Verification items for the finished model (mm, model axes). Face numbers are marked on the shaded views. A direction names the side the tool comes from. Round coordinates to 2 decimals unless told otherwise and drop trailing zeros. Write each loop counter-clockwise with the first axis right and the second up, starting at its lowest first coordinate (ties: lowest second). Pieces come first, ordered by that corner, then holes. Notation, with made-up numbers: (7.25, -29.75) - (21.25, -29.75) arc R33 ccw to (21.25, 2.25) - close; hole circle Ø6 at (7.25, -16.75). An arc over 180 degrees is marked (long way). Answer as a JSON object with one key per item and string values.
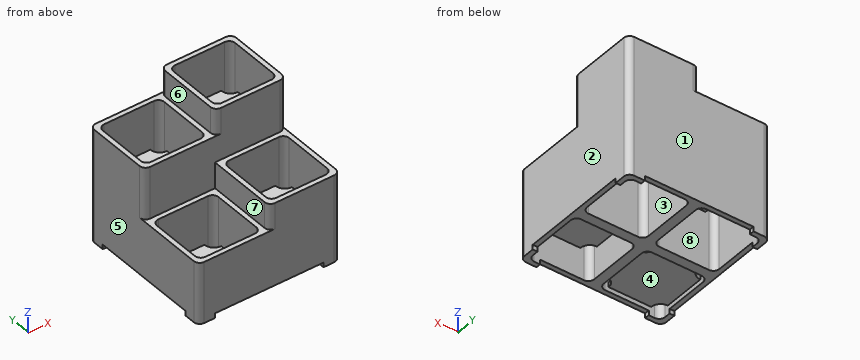
```python
from build123d import *

# Parameters (mm, degrees)
F0_W      = 4
F0_H      = 4
F1_DEPTH  = 48
F2_DEPTH  = 8
F3_DEPTH  = 70
F4_DEPTH  = 30
F0_H_2    = 23.163830772
F5_DEPTH  = 114
F6_DEPTH  = 74
F0_W_2    = 10.0586636961
F7_DEPTH  = 92
F8_DEPTH  = 52
F9_DEPTH  = 4
F10_DEPTH = 48
F11_DEPTH = 26
F12_DEPTH = 70
F13_DEPTH = 4
F14_R     = 5


with BuildPart() as f1:
    # F0 (on Top) → F1 (new body)
    with BuildSketch(Plane.XY):
        Polygon((-12, -4), (-4, -4), (-4, 0), (-56, 0), (-56, -4), (-48, -4), align=None)
        Polygon((-60, -56), (-56, -56), (-56, -48), (-56, -46), (-60, -46), align=None)
        Polygon((-4, -56), (0, -56), (0, -4), (-4, -4), (-4, -12), (-4, -48), align=None)
        with Locations((-2, -2)):
            Rectangle(F0_W, F0_H)
        Polygon((-60, 0), (-60, -46), (-56, -46), (-56, -16.2410065532), (-56, -12), (-56, -4), (-56, 0), align=None)
        Polygon((-46, -60), (0, -60), (0, -56), (-4, -56), (-12, -56), (-46, -56), align=None)
        Polygon((-56, -60), (-46, -60), (-46, -56), (-48, -56), (-56, -56), align=None)
        with Locations((-58, -58)):
            Rectangle(F0_W, F0_H)
    extrude(amount=F1_DEPTH)

    # F0 (on Top) → F2 (join)
    with BuildSketch(Plane.XY):
        with BuildLine():
            Line((-48, -56), (-46, -56))
            Line((-46, -56), (-12, -56))
            ThreePointArc((-12, -56), (-9.6568542495, -50.3431457505), (-4, -48))
            Line((-4, -48), (-4, -12))
            ThreePointArc((-4, -12), (-9.6568542495, -9.6568542495), (-12, -4))
            Line((-12, -4), (-48, -4))
            ThreePointArc((-48, -4), (-50.3431457505, -9.6568542495), (-56, -12))
            Line((-56, -12), (-56, -16.2410065532))
            Line((-56, -16.2410065532), (-56, -46))
            Line((-56, -46), (-56, -48))
            ThreePointArc((-56, -48), (-50.3431457505, -50.3431457505), (-48, -56))
        make_face()
    extrude(amount=F2_DEPTH)

    # F0 (on Top) → F3 (join)
    with BuildSketch(Plane.XY):
        Polygon((0, -4), (0, -56), (4, -56), (4, -48), (4, -12), (4, -4), align=None)
        with Locations((2, -2)):
            Rectangle(F0_W, F0_H)
        Polygon((56, -4), (56, 0), (4, 0), (4, -4), (12, -4), (48, -4), align=None)
        Polygon((56, -46), (60, -46), (60, 0), (56, 0), (56, -4), (56, -12), align=None)
        Polygon((0, -60), (46, -60), (46, -56), (12, -56), (4, -56), (0, -56), align=None)
        Polygon((56, -56), (60, -56), (60, -46), (56, -46), (56, -48), align=None)
        with Locations((58, -58)):
            Rectangle(F0_W, F0_H)
        Polygon((46, -60), (56, -60), (56, -56), (48, -56), (46, -56), align=None)
    extrude(amount=F3_DEPTH)

    # F0 (on Top) → F4 (join)
    with BuildSketch(Plane.XY):
        with BuildLine():
            Line((12, -56), (46, -56))
            Line((46, -56), (48, -56))
            ThreePointArc((48, -56), (50.3431457505, -50.3431457505), (56, -48))
            Line((56, -48), (56, -46))
            Line((56, -46), (56, -12))
            ThreePointArc((56, -12), (50.3431457505, -9.6568542495), (48, -4))
            Line((48, -4), (12, -4))
            ThreePointArc((12, -4), (9.6568542495, -9.6568542495), (4, -12))
            Line((4, -12), (4, -48))
            ThreePointArc((4, -48), (9.6568542495, -50.3431457505), (12, -56))
        make_face()
    extrude(amount=F4_DEPTH)

    # F0 (on Top) → F5 (join)
    with BuildSketch(Plane.XY):
        Polygon((0, 4), (4, 4), (4, 12), (4, 48), (4, 56), (0, 56), align=None)
        Polygon((0, 60), (0, 56), (4, 56), (12, 56), (46, 56), (46, 60), align=None)
        with Locations((58, 34.418084614)):
            Rectangle(F0_W, F0_H_2)
        Polygon((56, 0), (60, 0), (60, 22.836169228), (56, 22.836169228), (56, 12), (56, 4), align=None)
        Polygon((4, 0), (56, 0), (56, 4), (48, 4), (12, 4), (4, 4), align=None)
        with Locations((2, 2)):
            Rectangle(F0_W, F0_H)
        Polygon((48, 56), (56, 56), (56, 60), (46, 60), (46, 56), align=None)
        with Locations((58, 58)):
            Rectangle(F0_W, F0_H)
        Polygon((56, 46), (60, 46), (60, 56), (56, 56), (56, 48), align=None)
    extrude(amount=F5_DEPTH)

    # F0 (on Top) → F6 (join)
    with BuildSketch(Plane.XY):
        with BuildLine():
            Line((56, 12), (56, 22.836169228))
            Line((56, 22.836169228), (56, 46))
            Line((56, 46), (56, 48))
            ThreePointArc((56, 48), (50.3431457505, 50.3431457505), (48, 56))
            Line((48, 56), (46, 56))
            Line((46, 56), (12, 56))
            ThreePointArc((12, 56), (9.6568542495, 50.3431457505), (4, 48))
            Line((4, 48), (4, 12))
            ThreePointArc((4, 12), (9.6568542495, 9.6568542495), (12, 4))
            Line((12, 4), (48, 4))
            ThreePointArc((48, 4), (50.3431457505, 9.6568542495), (56, 12))
        make_face()
    extrude(amount=F6_DEPTH)

    # F0 (on Top) → F7 (join)
    with BuildSketch(Plane.XY):
        Polygon((-56, 0), (-4, 0), (-4, 4), (-12, 4), (-48, 4), (-56, 4), align=None)
        Polygon((-4, 4), (0, 4), (0, 56), (-4, 56), (-4, 48), (-4, 12), align=None)
        with Locations((-2, 2)):
            Rectangle(F0_W, F0_H)
        Polygon((-4, 56), (0, 56), (0, 60), (-35.9413363039, 60), (-35.9413363039, 56), (-12, 56), align=None)
        with Locations((-40.970668152, 58)):
            Rectangle(F0_W_2, F0_H)
        Polygon((-60, 0), (-56, 0), (-56, 4), (-56, 12), (-56, 46), (-60, 46), align=None)
        Polygon((-46, 56), (-46, 60), (-56, 60), (-56, 56), (-48, 56), align=None)
        with Locations((-58, 58)):
            Rectangle(F0_W, F0_H)
        Polygon((-60, 56), (-60, 46), (-56, 46), (-56, 48), (-56, 56), align=None)
    extrude(amount=F7_DEPTH)

    # F0 (on Top) → F8 (join)
    with BuildSketch(Plane.XY):
        with BuildLine():
            ThreePointArc((-12, 4), (-9.6568542495, 9.6568542495), (-4, 12))
            Line((-4, 12), (-4, 48))
            ThreePointArc((-4, 48), (-9.6568542495, 50.3431457505), (-12, 56))
            Line((-12, 56), (-35.9413363039, 56))
            Line((-35.9413363039, 56), (-46, 56))
            Line((-46, 56), (-48, 56))
            ThreePointArc((-48, 56), (-50.3431457505, 50.3431457505), (-56, 48))
            Line((-56, 48), (-56, 46))
            Line((-56, 46), (-56, 12))
            ThreePointArc((-56, 12), (-50.3431457505, 9.6568542495), (-48, 4))
            Line((-48, 4), (-12, 4))
        make_face()
    extrude(amount=F8_DEPTH)

    # F0 (on Top) → F9 (cut)
    with BuildSketch(Plane.XY):
        with BuildLine():
            Line((-48, -56), (-46, -56))
            Line((-46, -56), (-12, -56))
            ThreePointArc((-12, -56), (-9.6568542495, -50.3431457505), (-4, -48))
            Line((-4, -48), (-4, -12))
            ThreePointArc((-4, -12), (-9.6568542495, -9.6568542495), (-12, -4))
            Line((-12, -4), (-48, -4))
            ThreePointArc((-48, -4), (-50.3431457505, -9.6568542495), (-56, -12))
            Line((-56, -12), (-56, -16.2410065532))
            Line((-56, -16.2410065532), (-56, -46))
            Line((-56, -46), (-56, -48))
            ThreePointArc((-56, -48), (-50.3431457505, -50.3431457505), (-48, -56))
        make_face()
    extrude(amount=F9_DEPTH, mode=Mode.SUBTRACT)

    # F0 (on Top) → F10 (cut)
    with BuildSketch(Plane.XY):
        with BuildLine():
            ThreePointArc((-12, 4), (-9.6568542495, 9.6568542495), (-4, 12))
            Line((-4, 12), (-4, 48))
            ThreePointArc((-4, 48), (-9.6568542495, 50.3431457505), (-12, 56))
            Line((-12, 56), (-35.9413363039, 56))
            Line((-35.9413363039, 56), (-46, 56))
            Line((-46, 56), (-48, 56))
            ThreePointArc((-48, 56), (-50.3431457505, 50.3431457505), (-56, 48))
            Line((-56, 48), (-56, 46))
            Line((-56, 46), (-56, 12))
            ThreePointArc((-56, 12), (-50.3431457505, 9.6568542495), (-48, 4))
            Line((-48, 4), (-12, 4))
        make_face()
    extrude(amount=F10_DEPTH, mode=Mode.SUBTRACT)

    # F0 (on Top) → F11 (cut)
    with BuildSketch(Plane.XY):
        with BuildLine():
            Line((12, -56), (46, -56))
            Line((46, -56), (48, -56))
            ThreePointArc((48, -56), (50.3431457505, -50.3431457505), (56, -48))
            Line((56, -48), (56, -46))
            Line((56, -46), (56, -12))
            ThreePointArc((56, -12), (50.3431457505, -9.6568542495), (48, -4))
            Line((48, -4), (12, -4))
            ThreePointArc((12, -4), (9.6568542495, -9.6568542495), (4, -12))
            Line((4, -12), (4, -48))
            ThreePointArc((4, -48), (9.6568542495, -50.3431457505), (12, -56))
        make_face()
    extrude(amount=F11_DEPTH, mode=Mode.SUBTRACT)

    # F0 (on Top) → F12 (cut)
    with BuildSketch(Plane.XY):
        with BuildLine():
            Line((56, 12), (56, 22.836169228))
            Line((56, 22.836169228), (56, 46))
            Line((56, 46), (56, 48))
            ThreePointArc((56, 48), (50.3431457505, 50.3431457505), (48, 56))
            Line((48, 56), (46, 56))
            Line((46, 56), (12, 56))
            ThreePointArc((12, 56), (9.6568542495, 50.3431457505), (4, 48))
            Line((4, 48), (4, 12))
            ThreePointArc((4, 12), (9.6568542495, 9.6568542495), (12, 4))
            Line((12, 4), (48, 4))
            ThreePointArc((48, 4), (50.3431457505, 9.6568542495), (56, 12))
        make_face()
    extrude(amount=F12_DEPTH, mode=Mode.SUBTRACT)

    # F0 (on Top) → F13 (join)
    with BuildSketch(Plane.XY):
        Polygon((-46, 56), (-46, 60), (-56, 60), (-56, 56), (-48, 56), align=None)
        with Locations((-58, 58)):
            Rectangle(F0_W, F0_H)
        Polygon((-60, 56), (-60, 46), (-56, 46), (-56, 48), (-56, 56), align=None)
        Polygon((48, 56), (56, 56), (56, 60), (46, 60), (46, 56), align=None)
        with Locations((58, 58)):
            Rectangle(F0_W, F0_H)
        Polygon((56, 46), (60, 46), (60, 56), (56, 56), (56, 48), align=None)
        Polygon((56, -56), (60, -56), (60, -46), (56, -46), (56, -48), align=None)
        Polygon((46, -60), (56, -60), (56, -56), (48, -56), (46, -56), align=None)
        with Locations((58, -58)):
            Rectangle(F0_W, F0_H)
        Polygon((-60, -56), (-56, -56), (-56, -48), (-56, -46), (-60, -46), align=None)
        with Locations((-58, -58)):
            Rectangle(F0_W, F0_H)
        Polygon((-56, -60), (-46, -60), (-46, -56), (-48, -56), (-56, -56), align=None)
    extrude(amount=-F13_DEPTH)

    # F14
    f14_edges = [f1.edges().sort_by_distance(p)[0] for p in [
        (-60, 60, 44),
        (-60, 0, 70),
        (-60, -60, 22),
        (60, -60, 33),
        (0, -60, 59),
        (60, 60, 55),
        (0, 60, 103),
        (0, 0, 103),
        (60, 0, 92),
        (-4, 56, 46),
        (-4, 4, 46),
        (-56, 56, 44),
        (-56, 4, 46),
        (-56, -4, 24),
        (-4, -4, 24),
        (-4, -56, 24),
        (-56, -56, 22),
        (4, -56, 35),
        (4, -4, 35),
        (56, -4, 35),
        (56, -56, 33),
        (56, 4, 57),
        (56, 56, 55),
        (4, 56, 57),
        (4, 4, 57),
    ]]
    fillet(f14_edges, radius=F14_R)


solid = f1.part
```
Q1. Section check B-B, the plane z = 15. State how many separate pieces and enclosed holes the cut face has, then the cut area to 3 significant figures.
Geometry check:
{"separate pieces": "1", "enclosed holes": "4", "area": "3,650 mm2"}
Q2. Set-up check for the marked faces 4, 5, 6, 7 and 8: record each of +Z, -Z, +X, -X, +Y, -Y from which the full face is reachable in a straight line by a thin tool's end or side.
Geometry check:
{"face 4": "-Z", "face 5": "+Z, -Z, -X, +Y, -Y", "face 6": "+Z, -X, +Y, -Y", "face 7": "+Z, -X, -Y", "face 8": "none"}
Q3. Gauge pin test, flat ends, axial feed: P1, Ø5, axis at x = 19, y = -18.5, coming from the +Z side; P2, Ø2, axis at x = -59, z = -1.5, coming from the +Y side; P3, Ø12, axis at x = 30, y = -34.5, coming from the -Z side. Record the tip position at first contact, or that the pin passes through.
Geometry check:
{"P1": "stops at z = 30", "P2": "stops at y = 59", "P3": "stops at z = 26"}
Q4. Section check D-D, the plane y = 42. Record the cut outline in (x, z), then the cut area to 3 significant figures.
Geometry check:
{"outline": "(-60, 0) - (-56, 0) - (-56, 48) - (-4, 48) - (-4, 0) - (4, 0) - (4, 70) - (56, 70) - (56, 0) - (60, 0) - (60, 114) - (56, 114) - (56, 74) - (4, 74) - (4, 114) - (0, 114) - (0, 92) - (-4, 92) - (-4, 52) - (-56, 52) - (-56, 92) - (-60, 92) - close", "area": "2,060 mm2"}
Q5. Release check for a two-part mould opening along Y. For the marked faces 1, 2 and 3 record: released by +Y, released by -Y, zero draft, split by the parting line, or undercut.
Geometry check:
{"face 1": "released by +Y", "face 2": "zero draft", "face 3": "undercut"}
Q6. Section check C-C, the plane x = 32. Record the cut outline in (y, z).
Geometry check:
{"outline": "(-60, 0) - (-56, 0) - (-56, 26) - (-4, 26) - (-4, 0) - (4, 0) - (4, 70) - (56, 70) - (56, 0) - (60, 0) - (60, 114) - (56, 114) - (56, 74) - (4, 74) - (4, 114) - (0, 114) - (0, 70) - (-4, 70) - (-4, 30) - (-56, 30) - (-56, 70) - (-60, 70) - close"}
Q7. Material ranges on line 1 along Y through (x, z) = (40.5, 43); line 2 along Y through (x, z) = (-20.5, 87), recorded low to high. Write a range as [from, to].
Geometry check:
{"line 1": "y = [-60, -56], [-4, 4], [56, 60]", "line 2": "y = [0, 4], [56, 60]"}
Q8. Section check A-A, the plane y = -6. Record the cut outline in (x, z), then the cut area to 3 significant figures.
Geometry check:
{"outline": "(-60, 0) - (-55, 0) - (-55, 48) - (-60, 48) - close; (-48.25, 4) - (-11.75, 4) - (-11.75, 8) - (-48.25, 8) - close; (-5, 0) - (5, 0) - (5, 70) - (0, 70) - (0, 48) - (-5, 48) - close; (11.75, 26) - (48.25, 26) - (48.25, 30) - (11.75, 30) - close; (55, 0) - (60, 0) - (60, 70) - (55, 70) - close", "area": "1,470 mm2"}
